Can you work these out from the model? Positions are in its coordinate system, mm. Face numbers are marked on the shaded views. Give positions to 0.01 mm unless a question says otherwise; leave off trailing zeros. Loops run counter-clockwise (first coordinate to the right, second up) from the corner with the lowest first, then second, coordinate; pieces in that order, holes last. Notation, with made-up numbers: (2.25, 10.5) - (49.25, 10.5) arc R25 cw to (49.25, 45.5) - close; hole circle Ø8 at (66, 17). An arc over 180 degrees is marked (long way). Answer as a JSON object with one key per item and string values. Group by question number.
Item 1: Suppose I cut it at A-A on x = 0. Write out the boundary of the cut face in (y, z), and give its area (3 significant figures).
Item 2: Please list where these lines run through material, in increasing order: L1, parallel to Y at x = 0, z = 0.65; L2, parallel to Y at x = 15.5, z = 1.8; L3, parallel to X at y = -34.5, z = 2.4.
Item 3: Will these pins go through, and if not, where does the flat tip stop? pin 1 (4 mm diameter, centred on x = -38.5, y = -5, fed in from -Z); pin 2 (20 mm diameter, centred on x = 0, y = 0, fed in from +Z); pin 3 (1 mm diameter, centred on y = -14.5, z = 3, fed in from +X); pin 4 (3 mm diameter, centred on y = 15.5, z = 1, fed in from -X).
Item 4: Suppose I cut it at D-D on x = 10. Write out the boundary of the cut face in (y, z).
Item 5: Suppose I cut it at C-C on y = -32. Write out the boundary of the cut face in (x, z).
Item 6: Thinking about a two-plate mould opening in Y: for the marked faces 1 and 2, which applies, pulls with the +Y half, pulls with the -Y half, needs draft (parallel to the pull), parting line crosses it, or undercut?
Item 7: Suppose I cut it at B-B on y = 0. Write out the boundary of the cut face in (x, z), and give its area (3 significant figures).
Autodesk Inventor part; units mm, degrees
ref_plane "YZ Plane" through (0, 0, 0) normal (1, 0, 0) x (0, 1, 0)
ref_plane "XZ Plane" through (0, 0, 0) normal (0, 1, 0) x (-1, 0, 0)
ref_plane "XY Plane" through (0, 0, 0) normal (0, 0, 1) x (1, 0, 0)
sketch "Sketch1" plane through (0, 0, 0) normal (0, 0, 1) x (1, 0, 0)
  circle A0 centre (0, 0) radius 50
  circle A1 centre (0, 0) radius 3
  circle A2 centre (0, 45) radius 2.5
  circle A3 centre (-38.9711, 22.5) radius 2.5
  circle A4 centre (-38.9711, -22.5) radius 2.5
  circle A5 centre (0, -45) radius 2.5
  circle A6 centre (38.9711, -22.5) radius 2.5
  circle A7 centre (38.9711, 22.5) radius 2.5
  dimension "d0" = 100
  dimension "d1" = 6
  dimension "d2" = 5
  dimension "d3" = 45
  dimension "d6" = 360
extrude "Extrusion1" add sketch "Sketch1" along normal blind 5
sketch "Sketch2" plane through (0, 0, 5) normal (0, 0, 1) x (1, 0, 0)
  circle A0 centre (0, 0) radius 12.5
  dimension "d10" = 25
extrude "Extrusion2" cut sketch "Sketch2" against normal blind 2
sketch "Sketch3" plane through (0, 0, 5) normal (0, 0, 1) x (1, 0, 0)
  circle A0 centre (0, 0) radius 3
  circle A1 centre (0, 0) radius 25 construction
  circle A2 centre (0, 0) radius 40 construction
  line L0 (24, 7) -> (37.081, 15)
  line L1 (24, -7) -> (37.081, -15)
  line L2 (0, 0) -> (57.5693, 0) construction
  arc A3 (24, -7) -> (24, 7) centre (0, 0) ccw
  arc A4 (37.081, -15) -> (37.081, 15) centre (0, 0) ccw
  line L3 (5.9378, 24.2846) -> (5.5501, 39.6131)
  line L4 (18.0622, 17.2846) -> (31.5309, 24.6131)
  circle A5 centre (0, 0) radius 25 construction
  arc A6 (18.0622, 17.2846) -> (5.9378, 24.2846) centre (0, 0) ccw
  circle A7 centre (0, 0) radius 40 construction
  arc A8 (31.5309, 24.6131) -> (5.5501, 39.6131) centre (0, 0) ccw
  line L5 (-18.0622, 17.2846) -> (-31.5309, 24.6131)
  line L6 (-5.9378, 24.2846) -> (-5.5501, 39.6131)
  circle A9 centre (0, 0) radius 25 construction
  arc A10 (-5.9378, 24.2846) -> (-18.0622, 17.2846) centre (0, 0) ccw
  circle A11 centre (0, 0) radius 40 construction
  arc A12 (-5.5501, 39.6131) -> (-31.5309, 24.6131) centre (0, 0) ccw
  line L7 (-24, -7) -> (-37.081, -15)
  line L8 (-24, 7) -> (-37.081, 15)
  circle A13 centre (0, 0) radius 25 construction
  arc A14 (-24, 7) -> (-24, -7) centre (0, 0) ccw
  circle A15 centre (0, 0) radius 40 construction
  arc A16 (-37.081, 15) -> (-37.081, -15) centre (0, 0) ccw
  line L9 (-5.9378, -24.2846) -> (-5.5501, -39.6131)
  line L10 (-18.0622, -17.2846) -> (-31.5309, -24.6131)
  circle A17 centre (0, 0) radius 25 construction
  arc A18 (-18.0622, -17.2846) -> (-5.9378, -24.2846) centre (0, 0) ccw
  circle A19 centre (0, 0) radius 40 construction
  arc A20 (-31.5309, -24.6131) -> (-5.5501, -39.6131) centre (0, 0) ccw
  line L11 (18.0622, -17.2846) -> (31.5309, -24.6131)
  line L12 (5.9378, -24.2846) -> (5.5501, -39.6131)
  circle A21 centre (0, 0) radius 25 construction
  arc A22 (5.9378, -24.2846) -> (18.0622, -17.2846) centre (0, 0) ccw
  circle A23 centre (0, 0) radius 40 construction
  arc A24 (5.5501, -39.6131) -> (31.5309, -24.6131) centre (0, 0) ccw
  dimension "d13" = 50
  dimension "d14" = 80
  dimension "d15" = 15
  dimension "d16" = 7
  dimension "d19" = 360
extrude "Extrusion3" cut sketch "Sketch3" against normal through all contours L0 A4 L1 A3 | L3 A8 L4 A6 | L5 A12 L6 A10 | L7 A16 L8 A14 | L9 A20 L10 A18 | L11 A24 L12 A22
sketch "Sketch5" plane through (0, 0, 5) normal (0, 0, 1) x (1, 0, 0)
  line L0 (-15.5, -15.5) -> (15.5, -15.5) construction
  line L1 (15.5, -15.5) -> (15.5, 15.5) construction
  line L2 (15.5, 15.5) -> (-15.5, 15.5) construction
  line L3 (-15.5, 15.5) -> (-15.5, -15.5) construction
  line L4 (-15.5, -15.5) -> (15.5, 15.5) construction
  line L5 (15.5, -15.5) -> (-15.5, 15.5) construction
  circle A0 centre (-15.5, 15.5) radius 1.5
  circle A1 centre (15.5, 15.5) radius 1.5
  circle A2 centre (15.5, -15.5) radius 1.5
  circle A3 centre (-15.5, -15.5) radius 1.5
  point P0 (0, 0)
  dimension "d23" = 31
  dimension "d24" = 31
  dimension "d25" = 3
  dimension "d26" = 3
  dimension "d27" = 3
  dimension "d28" = 3
extrude "Extrusion4" cut sketch "Sketch5" against normal through all
equation "\"d29\" = d24"
properties part number "MC002" material "ABS Plastic"
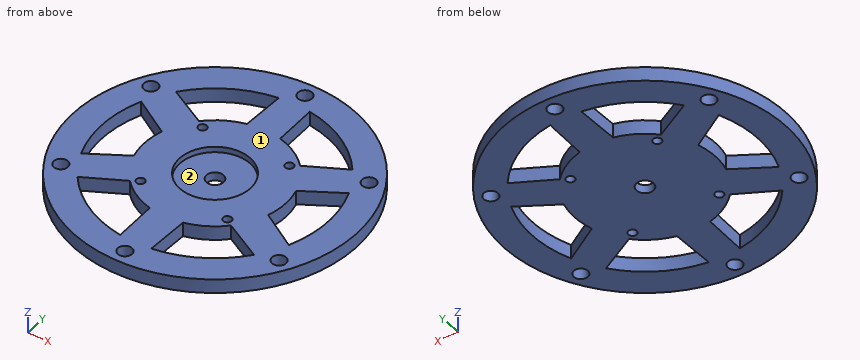
Worked out:
{
 "1": {"outline": "(-50, 0) - (-47.5, 0) - (-47.5, 5) - (-50, 5) - close; (-42.5, 0) - (-3, 0) - (-3, 3) - (-12.5, 3) - (-12.5, 5) - (-42.5, 5) - close; (3, 0) - (42.5, 0) - (42.5, 5) - (12.5, 5) - (12.5, 3) - (3, 3) - close; (47.5, 0) - (50, 0) - (50, 5) - (47.5, 5) - close", "area": "382 mm2"},
 "2": {"L1": "y = -50 to -47.5, -42.5 to -3, 3 to 42.5, 47.5 to 50", "L2": "y = -47.54 to -36.87, -19.62 to -17, -14 to 14, 17 to 19.62, 36.87 to 47.54", "L3": "x = -36.19 to -20.24, -5.68 to 5.68, 20.24 to 36.19"},
 "3": {"pin 1": "stops at z = 0", "pin 2": "stops at z = 3", "pin 3": "stops at x = 48", "pin 4": "stops at x = -48"},
 "4": {"outline": "(-48.99, 0) - (-38.73, 0) - (-38.73, 5) - (-48.99, 5) - close; (-22.91, 0) - (22.91, 0) - (22.91, 5) - (7.5, 5) - (7.5, 3) - (-7.5, 3) - (-7.5, 5) - (-22.91, 5) - close; (38.73, 0) - (48.99, 0) - (48.99, 5) - (38.73, 5) - close"},
 "5": {"outline": "(-38.42, 0) - (-24, 0) - (-24, 5) - (-38.42, 5) - close; (-5.74, 0) - (5.74, 0) - (5.74, 5) - (-5.74, 5) - close; (24, 0) - (38.42, 0) - (38.42, 5) - (24, 5) - close"},
 "6": {"face 1": "needs draft", "face 2": "undercut"},
 "7": {"outline": "(-50, 0) - (-40, 0) - (-40, 5) - (-50, 5) - close; (-25, 0) - (-3, 0) - (-3, 3) - (-12.5, 3) - (-12.5, 5) - (-25, 5) - close; (3, 0) - (25, 0) - (25, 5) - (12.5, 5) - (12.5, 3) - (3, 3) - close; (40, 0) - (50, 0) - (50, 5) - (40, 5) - close", "area": "282 mm2"}
}
